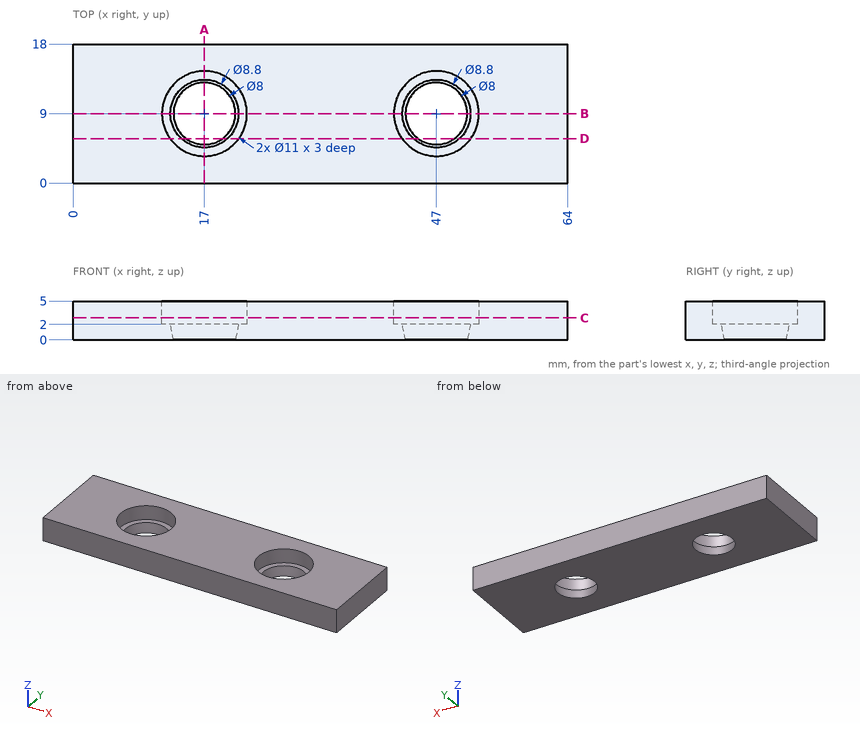
Design review of the part shown in the three views and the two pictorial views. Dimensions are in mm from the part's minimum x, y and z. Round coordinates to 2 decimals unless told otherwise and drop trailing zeros. Write each loop counter-clockwise with the first axis right and the second up, starting at its lowest first coordinate (ties: lowest second). Pieces come first, ordered by that corner, then holes. Notation, with made-up numbers: M 58,57 L 77,57 A18 cw 77,71 Z; hole C 15,-27 d1. An arc over 180 degrees is marked long. Use a Markdown table: item, result. Add a question column.
Q1. Insertion check: pin 1 (10 mm diameter, centred on x = 47, y = 9, fed in from +Z). The pin has a flat end and moves straight along its axis. Give the tip position at first contact, or say it passes through.
Q2. We need section B-B, the plane y = 9. State the section outline as (x, z) points.
Q3. We need section C-C, the plane z = 2.85. State the section outline as (x, y) points, plus the area to 3 significant figures.
Q4. To check wall thickness, follow line 1 (Y direction, x = 17, z = 2.6); line 2 (X direction, y = 9.25, z = 2.6); line 3 (Z direction, x = 21, y = 12.5). State the ranges of each line that lie inside material, in increasing order.
Q5. We need section D-D, the plane y = 5.75. Count the separate pieces of the cut face and the enclosed holes in it, plus the area to 4 significant figures.
Q6. We need section A-A, the plane x = 17. State the section outline as (y, z) points, plus the area to 3 significant figures.
Findings below:
| question | item | result |
|---|---|---|
| 1 | pin 1 | stops at z = 2 |
| 2 | outline | M 0,0 L 13,0 L 12.6,2 L 11.5,2 L 11.5,5 L 0,5 Z; M 21,0 L 43,0 L 42.6,2 L 41.5,2 L 41.5,5 L 22.5,5 L 22.5,2 L 21.4,2 Z; M 51,0 L 64,0 L 64,5 L 52.5,5 L 52.5,2 L 51.4,2 Z |
| 3 | outline | M 0,0 L 64,0 L 64,18 L 0,18 Z; hole C 17,9 d11; hole C 47,9 d11 |
| 3 | area | 962 mm² |
| 4 | line 1 | y = 0 to 3.5, 14.5 to 18 |
| 4 | line 2 | x = 0 to 11.51, 22.49 to 41.51, 52.49 to 64 |
| 4 | line 3 | z = 0 to 2 |
| 5 | separate pieces | 3 |
| 5 | enclosed holes | 0 |
| 5 | area | 245.5 mm² |
| 6 | outline | M 0,0 L 5,0 L 4.6,2 L 3.5,2 L 3.5,5 L 0,5 Z; M 13,0 L 18,0 L 18,5 L 14.5,5 L 14.5,2 L 13.4,2 Z |
| 6 | area | 40.2 mm² |
